Could you check a few things on this model? Use its own coordinates, in mm. Face numbers are marked on the shaded views. A direction names the side the tool comes from. Round coordinates to 2 decimals unless told otherwise and drop trailing zeros. Write each loop counter-clockwise with the first axis right and the second up, starting at its lowest first coordinate (ties: lowest second). Pieces come first, ordered by that corner, then holes. Notation, with made-up numbers: M -26,64.25 L -2,64.25 A12 ccw -2,72.25 Z; hole C 57.5,-29.5 d7. An arc over 180 degrees is marked long. One line per item, written item: value. Start each with the question number.
(1) Which directions (+Z, -Z, +X, -X, +Y, -Y) give clear straight access to the entire face, cutting with the end or side of a thin tool? Please do the marked faces 5, 6, 7, 8 and 9.
(2) I'm going to push flat-ended pins straight in: pin 1 Ø1.5 at (x, z) = (-2.5, -4.5) entering from -Y; pin 2 Ø1.2 at (x, z) = (9.5, 0) entering from -Y; pin 3 Ø4 at (x, y) = (4, -13) entering from +Z; pin 4 Ø6 at (x, z) = (1, -5) entering from -Y. Where does each tip first touch, or does it pass through?
(3) Thinking about a two-plate mould opening in Y: for the marked faces 1, 2, 3 and 4, which applies, released by +Y, released by -Y, zero draft, split by the parting line, or undercut?
(4) I want a section at A-A on z = 0. Please give me the cut outline in (x, y), and give its area (3 significant figures).
(5) I want a section at D-D on x = 8.25. Please give me the cut outline in (y, z), and give its area (3 significant figures).
(6) I want a section at C-C on x = -5.75. Please give me the cut outline in (y, z).
(7) If I drill on L1, parallel to Y at x = 6.25, z = 1; L2, parallel to Y at x = 5.5, z = 2.5; L3, parallel to Y at x = 11.25, z = -1.75, over which ranges is the centre line in solid material (lowest first)?
(8) I want a section at B-B on z = 5.5. Please give me the cut outline in (x, y), and give its area (3 significant figures).
```python
from build123d import *

# Parameters (mm, degrees)
SKETCH1_R                = 6.9469
BOSS_EXTRUDE1_DEPTH      = 4.22
SKETCH2_R                = 3.51
BOSS_EXTRUDE2_DEPTH      = 17.46
BOSS_EXTRUDE3_DEPTH      = 14.5
BOSS_EXTRUDE3_DEPTH_BACK = 7.5


with BuildPart() as part:
    # Sketch1 → Boss-Extrude1 (new body)
    with BuildSketch(Plane(origin=(0, 0, 0), x_dir=(1, 0, 0), z_dir=(0, 1, 0))):
        with Locations(Location((0, 0, 0), (0, 0, 270))):
            Circle(SKETCH1_R)
    extrude(amount=BOSS_EXTRUDE1_DEPTH)

    # Sketch2 → Boss-Extrude2 (add)
    with BuildSketch(Plane(origin=(0, 0, 0), x_dir=(-1, 0, 0), z_dir=(0, -1, 0))):
        with Locations(Location((0, 0, 0), (0, 0, 90))):
            Circle(SKETCH2_R)
    extrude(amount=BOSS_EXTRUDE2_DEPTH)

    # Sketch3 → Boss-Extrude3 (add, two sides: drawn at the far end of the back side and taken through both)
    with BuildSketch(Plane(origin=(0, 0, 0), x_dir=(0, 0, -1), z_dir=(1, 0, 0)).offset(-BOSS_EXTRUDE3_DEPTH_BACK)):
        with BuildLine():
            Line((-6.249999984, -10.41), (-6.75, -10.41))
            ThreePointArc((-6.75, -10.41), (-4.807849454, -13.931255454), (-2, -16.81))
            Line((-2, -16.81), (2, -16.81))
            ThreePointArc((2, -16.81), (4.807849454, -13.931255454), (6.75, -10.41))
            Line((6.75, -10.41), (6.249999984, -10.41))
            Line((6.249999984, -10.41), (4.3, -10.41))
            Line((4.3, -10.41), (3.5, -9.61))
            Line((3.5, -9.61), (-3.5, -9.61))
            Line((-3.5, -9.61), (-4.3, -10.41))
            Line((-4.3, -10.41), (-6.249999984, -10.41))
        make_face()
    extrude(amount=BOSS_EXTRUDE3_DEPTH + BOSS_EXTRUDE3_DEPTH_BACK)


solid = part.part
```
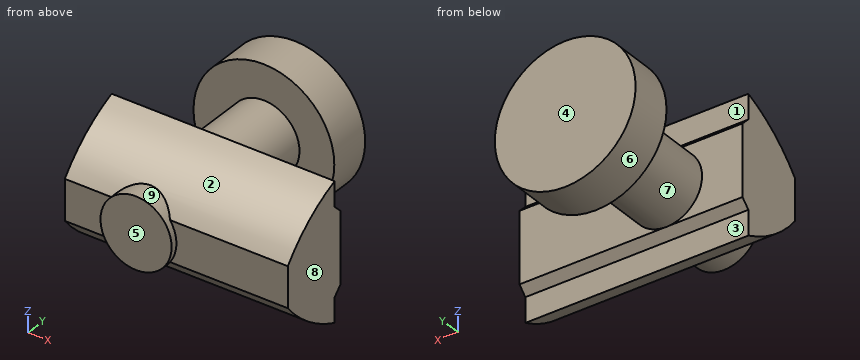
Found:
1. face 5: +Z, -Z, +X, -X, -Y
1. face 6: +Y
1. face 7: none
1. face 8: +Z, -Z, +X, +Y, -Y
1. face 9: -Y
2. pin 1: stops at y = -15.2
2. pin 2: stops at y = -16.81
2. pin 3: stops at z = 6.51
2. pin 4: stops at y = -17.46
3. face 1: undercut
3. face 2: released by -Y
3. face 3: undercut
3. face 4: released by +Y
4. outline: M -7.5,-16.81 L -3.51,-16.81 L -3.51,-17.46 L 3.51,-17.46 L 3.51,-16.81 L 14.5,-16.81 L 14.5,-9.61 L 3.51,-9.61 L 3.51,0 L 6.95,0 L 6.95,4.22 L -6.95,4.22 L -6.95,0 L -3.51,0 L -3.51,-9.61 L -7.5,-9.61 Z
4. area: 289 mm²
5. outline: M -16.81,-2 A15 ccw -10.41,-6.75 L -10.41,-4.3 L -9.61,-3.5 L -9.61,3.5 L -10.41,4.3 L -10.41,6.75 A15 ccw -16.81,2 Z
5. area: 68.0 mm²
6. outline: M -16.81,-2 A15 ccw -10.41,-6.75 L -10.41,-4.3 L -9.61,-3.5 L -9.61,3.5 L -10.41,4.3 L -10.41,6.75 A15 ccw -16.81,2 Z; M 0,-3.9 L 4.22,-3.9 L 4.22,3.9 L 0,3.9 Z
7. L1: y = -16.81 to -9.61, 0 to 4.22
7. L2: y = -16.4 to -9.61, 0 to 4.22
7. L3: y = -16.81 to -9.61
8. outline: M -7.5,-12.91 L 14.5,-12.91 L 14.5,-10.41 L -7.5,-10.41 Z; M -4.24,0 L 4.24,0 L 4.24,4.22 L -4.24,4.22 Z
8. area: 90.9 mm²
